Design review of the part built by this model. Coordinates are the model's own, in mm. Give positions to 0.01 mm unless a question says otherwise; leave off trailing zeros. Write each loop counter-clockwise with the first axis right and the second up, starting at its lowest first coordinate (ties: lowest second). Pieces come first, ordered by that corner, then holes.
```python
from build123d import *

# Parameters (mm, degrees)
BOSS_EXTRUDE1_DEPTH = 3.6
SKETCH3_R           = 2.25
CUT_EXTRUDE1_DEPTH  = 10


with BuildPart() as part:
    # Sketch1 → Boss-Extrude1 (new body)
    with BuildSketch(Plane.XY):
        Polygon((3, 408), (-12.5, 408), (-12.5, 405), (-22.5, 405), (-22.5, 408), (-32.5, 408), (-32.5, 405), (-42.5, 405), (-42.5, 408), (-52.5, 408), (-52.5, 405), (-62.5, 405), (-62.5, 408), (-72.5, 408), (-72.5, 405), (-82.5, 405), (-82.5, 408), (-92.5, 408), (-92.5, 405), (-102.5, 405), (-102.5, 408), (-112.5, 408), (-112.5, 405), (-122.5, 405), (-122.5, 408), (-132.5, 408), (-132.5, 405), (-142.5, 405), (-142.5, 408), (-152.5, 408), (-152.5, 405), (-162.5, 405), (-162.5, 408), (-178, 408), (-178, 397.5), (-175, 397.5), (-175, 387.5), (-178, 387.5), (-178, 377.5), (-175, 377.5), (-175, 367.5), (-178, 367.5), (-178, 357.5), (-175, 357.5), (-175, 347.5), (-178, 347.5), (-178, 337.5), (-175, 337.5), (-175, 327.5), (-178, 327.5), (-178, 317.5), (-175, 317.5), (-175, 307.5), (-178, 307.5), (-178, 297.5), (-175, 297.5), (-175, 287.5), (-178, 287.5), (-178, 277.5), (-175, 277.5), (-175, 267.5), (-178, 267.5), (-178, 257.5), (-175, 257.5), (-175, 0), (-175, -23), (-178, -23), (-178, -33), (-175, -33), (-175, -43), (-178, -43), (-178, -53), (-175, -53), (-175, -63), (-178, -63), (-178, -73), (3, -73), (3, -63), (0, -63), (0, -53), (3, -53), (3, -43), (0, -43), (0, -33), (3, -33), (3, -23), (0, -23), (0, 0), (0, 257.5), (3, 257.5), (3, 267.5), (0, 267.5), (0, 277.5), (3, 277.5), (3, 287.5), (0, 287.5), (0, 297.5), (3, 297.5), (3, 307.5), (0, 307.5), (0, 317.5), (3, 317.5), (3, 327.5), (0, 327.5), (0, 337.5), (3, 337.5), (3, 347.5), (0, 347.5), (0, 357.5), (3, 357.5), (3, 367.5), (0, 367.5), (0, 377.5), (3, 377.5), (3, 387.5), (0, 387.5), (0, 397.5), (3, 397.5), align=None)
    extrude(amount=BOSS_EXTRUDE1_DEPTH)

    # Sketch3 → Cut-Extrude1 (cut)
    with BuildSketch(Plane.XY.offset(3.6)):
        with Locations((-142.5, 365)):
            Circle(SKETCH3_R)
        with Locations((-32.5, 69.049357195)):
            Circle(SKETCH3_R)
        with Locations((-32.5, 99.549357195)):
            Circle(SKETCH3_R)
        with Locations((-142.5, 69.049357195)):
            Circle(SKETCH3_R)
        with Locations((-142.5, 99.549357195)):
            Circle(SKETCH3_R)
        with Locations((-142.5, 156.719761425)):
            Circle(SKETCH3_R)
        with Locations((-32.5, 156.719761425)):
            Circle(SKETCH3_R)
        with Locations((-32.5, 202.219761425)):
            Circle(SKETCH3_R)
        with Locations((-142.5, 202.219761425)):
            Circle(SKETCH3_R)
        with Locations((-32.5, 365)):
            Circle(SKETCH3_R)
        with Locations((-32.5, 395)):
            Circle(SKETCH3_R)
        with Locations((-142.5, 395)):
            Circle(SKETCH3_R)
    extrude(amount=-CUT_EXTRUDE1_DEPTH, mode=Mode.SUBTRACT)


solid = part.part
```
(1) Consider section A-A, the plane y = 123.5. Give the boundary of the cut face in (x, z).
Resolved:
outline: (-175, 0) - (0, 0) - (0, 3.6) - (-175, 3.6) - close
(2) Clearance check with flat-ended pins moving along their axes: P1, Ø1, axis at y = 117.5, z = 0.5, coming from the +X side; P2, Ø1, axis at y = 205, z = 1.5, coming from the -X side; P3, Ø4, axis at x = -142.5, y = 99.55, coming from the +Z side; P4, Ø5, axis at x = -133.5, y = 153, coming from the -Z side. State where each tip first meets the part, or that it passes through.
Resolved:
P1: stops at x = 0
P2: stops at x = -175
P3: passes through
P4: stops at z = 0
(3) To check wall thickness, follow L1, parallel to X at y = 365, z = 1.65; L2, parallel to X at y = 68, z = 2.9; L3, parallel to X at y = 290, z = 0.55. State the ranges of each line that lie inside material, in increasing order.
Resolved:
L1: x = -178 to -144.75, -140.25 to -34.75, -30.25 to 3
L2: x = -175 to -144.49, -140.51 to -34.49, -30.51 to 0
L3: x = -175 to 0
(4) Consider section B-B, the plane z = 2.35. Give the number of separate pieces and of enclosed holes in the cut face, then the cut area to 3 significant figures.
Resolved:
separate pieces: 1
enclosed holes: 12
area: 84,400 mm2
